Answer from the drawing. Dimensions are ordinates in mm from the lowest x, y and z of the part. A direction names the side the tool comes from. Coordinates: 2 decimals unless noted, no trailing zeros. Loops run counter-clockwise (first coordinate to the right, second up) from the corner with the lowest first, then second, coordinate; pieces in that order, holes last.
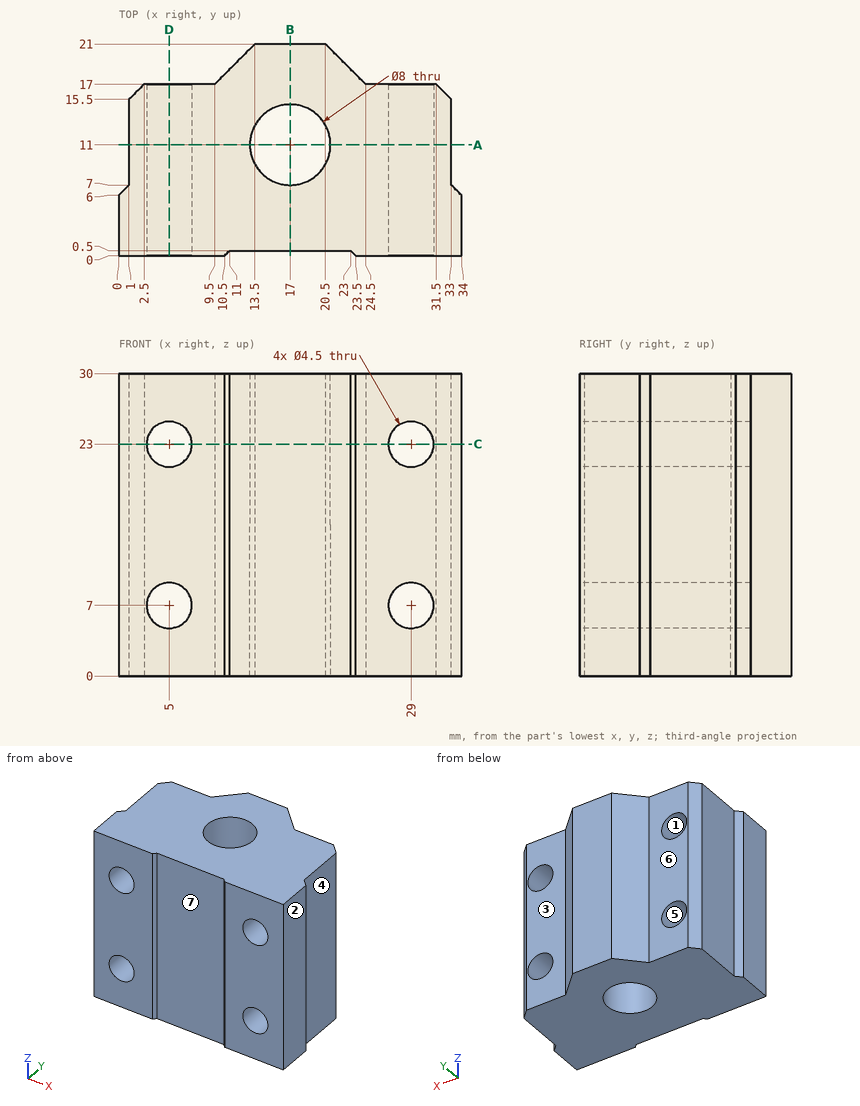
Item 1: Given pin 1 (9.5 mm diameter, centred on x = 14.5, z = 21.5, fed in from -Y); pin 2 (7 mm diameter, centred on y = 13, z = 14.5, fed in from +X); pin 3 (1.5 mm diameter, centred on y = 8, z = 9, fed in from -X); pin 4 (5.5 mm diameter, centred on x = 28, z = 19, fed in from +Y), each flat-ended and moving along its own axis, determine where each tip first touches the part or whether it passes through.
Numbers:
pin 1: stops at y = 0
pin 2: stops at x = 33
pin 3: stops at x = 1
pin 4: stops at y = 17
Item 2: A cutting plane is placed at A-A on y = 11. Determine the outline of the cut face in (x, z), then the cut area to 3 significant figures.
Numbers:
outline: (1, 0) - (13, 0) - (13, 30) - (1, 30) - close; (21, 0) - (33, 0) - (33, 30) - (21, 30) - close; hole circle Ø4.5 at (5, 7); hole circle Ø4.5 at (5, 23); hole circle Ø4.5 at (29, 7); hole circle Ø4.5 at (29, 23)
area: 656 mm2
Item 3: A cutting plane is placed at C-C on z = 23. Determine the outline of the cut face in (x, y), then the cut area to 3 significant figures.
Numbers:
outline: (0, 0) - (2.75, 0) - (2.75, 17) - (2.5, 17) - (1, 15.5) - (1, 7) - (0, 6) - close; (7.25, 0) - (10.5, 0) - (11, 0.5) - (23, 0.5) - (23.5, 0) - (26.75, 0) - (26.75, 17) - (24.5, 17) - (20.5, 21) - (13.5, 21) - (9.5, 17) - (7.25, 17) - close; (31.25, 0) - (34, 0) - (34, 6) - (33, 7) - (33, 15.5) - (31.5, 17) - (31.25, 17) - close; hole circle Ø8 at (17, 11)
area: 389 mm2
Item 4: A cutting plane is placed at B-B on x = 17. Determine the outline of the cut face in (y, z).
Numbers:
outline: (0.5, 0) - (7, 0) - (7, 30) - (0.5, 30) - close; (15, 0) - (21, 0) - (21, 30) - (15, 30) - close
Item 5: Find the intervals of material crossed by line 1 along X through (y, z) = (4.25, 23); line 2 along Z through (x, y) = (29, 13.5); line 3 along Y through (x, z) = (17, 6.75), in increasing order.
Numbers:
line 1: x = 0 to 2.75, 7.25 to 26.75, 31.25 to 34
line 2: z = 0 to 4.75, 9.25 to 20.75, 25.25 to 30
line 3: y = 0.5 to 7, 15 to 21
Item 6: Which of the six approach directions +Z, -Z, +X, -X, +Y, -Y give full straight-line access (tool end or side, diameter ignored) to the marked faces 4, 5, 6 and 7?
Numbers:
face 4: +Z, -Z, +X, +Y
face 5: +Y, -Y
face 6: +Z, -Z, -X, +Y
face 7: +Z, -Z, -Y
Item 7: Determine the mould class of the marked faces 1, 2 and 3 for opening direction X: released by +X, released by -X, zero draft, split by the parting line, or undercut.
Numbers:
face 1: undercut
face 2: released by +X
face 3: zero draft
Item 8: A cutting plane is placed at D-D on x = 5. Determine the outline of the cut face in (y, z).
Numbers:
outline: (0, 0) - (17, 0) - (17, 4.75) - (0, 4.75) - close; (0, 9.25) - (17, 9.25) - (17, 20.75) - (0, 20.75) - close; (0, 25.25) - (17, 25.25) - (17, 30) - (0, 30) - close
